from build123d import *

# Parameters (mm, degrees)
SKETCH3_R                   = 3.81
DOWELSUPPORT_DEPTH          = 1.27
SKETCH5_W                   = 6.35
SKETCH5_H                   = 44.45
SLIDERDOWELSUPPORT_DEPTH    = 1.27
LATERALSUPPORT_DEPTH        = 1.27
SKETCH8_W                   = 6.35
SKETCH8_H                   = 3
TABSUPPORT_DEPTH            = 1.27
STRINGDOWELSUPPORT_START    = -1.27
STRINGDOWELSUPPORT_DEPTH    = 5.08
INTERSUPPORT_DEPTH          = 1.27
SKETCH10_W                  = 6.35
SKETCH10_H                  = 3
TABBASE_DEPTH               = 1.27
SKETCH12_W                  = 6.35
SKETCH12_H                  = 3
TABDRAFT_DEPTH              = 1.73
TABDRAFT_DRAFT              = 5
TABDRAFT_PROFILE_2_DEPTH    = 1.73
TABDRAFT_PROFILE_2_DRAFT    = 5
STRINGDOWELHOLES_DEPTH      = 48.469574456
STRINGDOWELHOLES_DEPTH_BACK = 1.524
SKETCH14_R                  = 1.690500048
PULLEYDOWELHOLE_DEPTH       = 2.54


with BuildPart() as part:
    # Sketch3 → DowelSupport (new, symmetric)
    with BuildSketch(Plane(origin=(0, 0, 0), x_dir=(0, 0, -1), z_dir=(1, 0, 0))):
        with Locations((0, 37.30625)):
            Circle(SKETCH3_R)
    extrude(amount=DOWELSUPPORT_DEPTH, both=True)

    # Sketch8 → TabSupport (add, symmetric)
    with BuildSketch(Plane(origin=(0, 0, 0), x_dir=(0, 0, -1), z_dir=(1, 0, 0))):
        with Locations((0, 34.29)):
            Rectangle(SKETCH8_W, SKETCH8_H)
        with Locations((-12.7, 34.29)):
            Rectangle(SKETCH8_W, SKETCH8_H)
    extrude(amount=TABSUPPORT_DEPTH, both=True)


with BuildPart() as body_2:
    # Sketch5 → SliderDowelSupport (new, symmetric)
    with BuildSketch(Plane(origin=(0, 0, 0), x_dir=(0, 0, -1), z_dir=(1, 0, 0))):
        Rectangle(SKETCH5_W, SKETCH5_H)
    extrude(amount=SLIDERDOWELSUPPORT_DEPTH, both=True)



with BuildPart() as body_3:
    # Sketch6 → LateralSupport (new, symmetric)
    with BuildSketch(Plane(origin=(0, 0, 0), x_dir=(0, 0, -1), z_dir=(1, 0, 0))):
        Polygon((7.392863577, 39.741434671), (5.805363577, 42.491065329), (8.403439788, 43.991065329), (9.990939788, 41.241434671), align=None)
    extrude(amount=LATERALSUPPORT_DEPTH, both=True)


with BuildPart() as tabsupport_piece_1:
    # of the separate pieces the step leaves, piece 1, a body of its own (tabsupport_pieces)
    add(part.part.solids().sort_by_distance((1.27, 35.200193258, 3.175))[0])


with BuildPart() as tabsupport_piece_2:
    # of the separate pieces the step leaves, piece 2, a body of its own (tabsupport_pieces)
    add(part.part.solids().sort_by_distance((-1.27, 32.79, 9.525))[0])

    # Sketch15 → StringDowelSupport (add)
    with BuildSketch(Plane(origin=(0, 0, 0), x_dir=(0, 0, -1), z_dir=(1, 0, 0)).offset(STRINGDOWELSUPPORT_START)):
        with BuildLine():
            Line((-14.4145, 36.298), (-10.9855, 36.298))
            ThreePointArc((-10.9855, 36.298), (-8.4455, 33.758), (-10.9855, 31.218))
            Line((-10.9855, 31.218), (-14.4145, 31.218))
            ThreePointArc((-14.4145, 31.218), (-16.9545, 33.758), (-14.4145, 36.298))
        make_face()
    extrude(amount=STRINGDOWELSUPPORT_DEPTH)


with BuildPart() as body_2_1:
    add(body_2.part)

    add(body_3.part)  # InterSupport merges body 3

    add(tabsupport_piece_1.part)  # InterSupport merges TabSupport piece 1

    add(tabsupport_piece_2.part)  # InterSupport merges TabSupport piece 2
    # Sketch7 → InterSupport (add, symmetric)
    with BuildSketch(Plane(origin=(0, 0, 0), x_dir=(0, 0, -1), z_dir=(1, 0, 0))):
        Polygon((-15.691284512, 32.81461378), (-3.175, 15.875), (-3.175, 22.225), (3.175, 22.225), (3.175, 32.79), (0.989321966, 34.625476176), (-0.989321966, 39.987023824), (-10.9855, 36.298), (-14.4145, 36.298), align=None)
        Polygon((5.170363577, 43.590917591), (8.027863577, 38.641582409), (1.42875, 34.831582409), (-1.42875, 39.780917591), align=None)
    extrude(amount=INTERSUPPORT_DEPTH, both=True)

    # Sketch10 → TabBase (add)
    with BuildSketch(Plane.ZY.offset(1.27)):
        with Locations((0, 34.29)):
            Rectangle(SKETCH10_W, SKETCH10_H)
        with Locations((12.7, 34.29)):
            Rectangle(SKETCH10_W, SKETCH10_H)
    extrude(amount=TABBASE_DEPTH)


with BuildPart() as tabdraft_tool:
    # Sketch12 → TabDraft (with draft: the straight prism first)
    with BuildSketch(Plane.ZY.offset(2.54)):
        with Locations((0, 34.29)):
            Rectangle(SKETCH12_W, SKETCH12_H)
    extrude(amount=TABDRAFT_DEPTH)
    # TabDraft: the draft: its side faces are tilted about the plane it starts from
    tabdraft_sides = [tabdraft_tool.faces().sort_by_distance(p)[0] for p in [
        (-3.405, 34.29, 3.175),
        (-3.405, 35.79, 0),
        (-3.405, 34.29, -3.175),
        (-3.405, 32.79, 0),
    ]]
    draft(tabdraft_sides, Plane.ZY.offset(2.54), TABDRAFT_DRAFT)


with BuildPart() as body_2_2:
    add(body_2_1.part)

    # TabDraft: add tabdraft_tool
    add(tabdraft_tool.part)


with BuildPart() as tabdraft_profile_2_tool:
    # Sketch12 → TabDraft profile 2 (with draft: the straight prism first)
    with BuildSketch(Plane.ZY.offset(2.54)):
        with Locations((12.7, 34.29)):
            Rectangle(SKETCH12_W, SKETCH12_H)
    extrude(amount=TABDRAFT_PROFILE_2_DEPTH)
    # TabDraft profile 2: the draft: its side faces are tilted about the plane it starts from
    tabdraft_profile_2_sides = [tabdraft_profile_2_tool.faces().sort_by_distance(p)[0] for p in [
        (-3.405, 34.29, 9.525),
        (-3.405, 32.79, 12.7),
        (-3.405, 34.29, 15.875),
        (-3.405, 35.79, 12.7),
    ]]
    draft(tabdraft_profile_2_sides, Plane.ZY.offset(2.54), TABDRAFT_PROFILE_2_DRAFT)


with BuildPart() as body_2_3:
    add(body_2_2.part)

    # TabDraft profile 2: add tabdraft_profile_2_tool
    add(tabdraft_profile_2_tool.part)

    # Sketch16 → StringDowelHoles (cut, two sides: drawn at the far end of the back side and taken through both)
    with BuildSketch(Plane(origin=(1.27, 0, 0), x_dir=(0, 0, -1), z_dir=(1, 0, 0)).offset(-STRINGDOWELHOLES_DEPTH_BACK)):
        with BuildLine():
            Line((-12.905478326, 32.996), (-12.494521674, 32.996))
            ThreePointArc((-12.494521674, 32.996), (-9.294999952, 33.758), (-12.494521674, 34.52))
            Line((-12.494521674, 34.52), (-12.905478326, 34.52))
            ThreePointArc((-12.905478326, 34.52), (-16.105000048, 33.758), (-12.905478326, 32.996))
        make_face()
    extrude(amount=STRINGDOWELHOLES_DEPTH + STRINGDOWELHOLES_DEPTH_BACK, mode=Mode.SUBTRACT)

    # Sketch14 → PulleyDowelHole (cut)
    with BuildSketch(Plane(origin=(1.27, 0, 0), x_dir=(0, 0, -1), z_dir=(1, 0, 0))):
        with Locations((0, 37.30625)):
            Circle(SKETCH14_R)
    extrude(amount=-PULLEYDOWELHOLE_DEPTH, mode=Mode.SUBTRACT)

    # Mirror1: body 2 across plane


with BuildPart() as body_2_4:
    add(body_2_3.part)
    add(body_2_3.part.mirror(Plane.ZX))


solid = body_2_4.part
Design review of the part built by this model. Coordinates are the model's own, in mm. A direction names the side the tool comes from. Round coordinates to 2 decimals unless told otherwise and drop trailing zeros. Write each loop counter-clockwise with the first axis right and the second up, starting at its lowest first coordinate (ties: lowest second). Pieces come first, ordered by that corner, then holes. Notation, with made-up numbers: (-39.75, -6.75) - (11.25, -6.75) arc R11 ccw to (11.25, -0.75) - close; hole circle Ø4 at (11, 5). An arc over 180 degrees is marked (long way). Use a Markdown table: item, result. Add a question column.
1. We need section D-D (y = 12.5). State the section outline as (x, z) points (3 decimals).
2. We need section A-A (x = 2.25). State the section outline as (y, z) points.
3. We need section B-B (z = 0). State the section outline as (x, y) points.
4. Clearance check with flat-ended pins moving along their axes: pin 1 (0.6 mm diameter, centred on x = -2, y = -34.5, fed in from +Z) (3 decimals); pin 2 (3 mm diameter, centred on x = 0, y = 7.5, fed in from +Z) (3 decimals); pin 3 (1 mm diameter, centred on x = -2, z = 12, fed in from -Y). State where each tip first meets the part, or that it passes through.
5. For faces 1 (the face through (-3.393, -32.865, 12.656)), 2 (the face through (3, -31.218, 13)), 3 (the face through (0.02, -40.5, -8.71)), 4 (the face through (-3.4, -34.3, 3.1)), 5 (the face through (0.02, 23.65, 8.92)), list the 3-axis set-ups (+Z, -Z, +X, -X, +Y, -Y) from which the entire face can be reached by the end or side of a thin tool; tool diameter is ignored.
6. Mouldability with a two-part tool opening along Z and no side actions: class faces 6 (the face through (1.75, 33.821, 16.104)), 7 (the face through (-3.4, -34.3, 9.6)), 8 (the face through (-3.393, 32.865, 12.656)), 9 (the face through (2.522, -33.814, 8.446)) as +Z half, -Z half, draft (parallel to the pull), parting line (faces both ways), or undercut.
7. Wall thickness on probe 1 along Y at (x, z) = (0.3, 0); probe 2 along Z at (x, y) = (-2.75, -34); probe 3 along X at (y, z) = (27.5, -2): over which ranges is each line inside the solid? List them lowest first.
8. We need section C-C (z = 4.75). State the section outline as (x, y) points.
Output:
| question | item | result |
|---|---|---|
| 1 | outline | (-1.27, -3.175) - (1.27, -3.175) - (1.27, 3.175) - (-1.27, 3.175) - close |
| 2 | outline | (-36.3, 10.99) arc R2.54 ccw to (-31.22, 10.99) - (-31.22, 14.41) arc R2.54 ccw to (-36.3, 14.41) - close; (31.22, 10.99) arc R2.54 ccw to (36.3, 10.99) - (36.3, 14.41) arc R2.54 ccw to (31.22, 14.41) - close; hole (-34.52, 12.49) arc R1.69 ccw (long way) to (-33, 12.49) - (-33, 12.91) arc R1.69 ccw (long way) to (-34.52, 12.91) - close; hole (33, 12.49) arc R1.69 ccw (long way) to (34.52, 12.49) - (34.52, 12.91) arc R1.69 ccw (long way) to (33, 12.91) - close |
| 3 | outline | (-4.27, -35.64) - (-2.54, -35.79) - (-1.27, -35.79) - (-1.27, -35.62) - (1.27, -35.62) - (1.27, 35.62) - (-1.27, 35.62) - (-1.27, 35.79) - (-2.54, 35.79) - (-4.27, 35.64) - (-4.27, 32.94) - (-2.54, 32.79) - (-1.27, 32.79) - (-1.27, -32.79) - (-2.54, -32.79) - (-4.27, -32.94) - close; (-1.27, -41.12) - (1.27, -41.12) - (1.27, -39) - (-1.27, -39) - close; (-1.27, 39) - (1.27, 39) - (1.27, 41.12) - (-1.27, 41.12) - close |
| 4 | pin 1 | stops at z = 15.875 |
| 4 | pin 2 | stops at z = 3.175 |
| 4 | pin 3 | stops at y = -35.79 |
| 5 | face 1 | +Z, -Z, -X |
| 5 | face 2 | +Z, -Z, +X |
| 5 | face 3 | -Z, +X, -X |
| 5 | face 4 | -X, +Y, -Y |
| 5 | face 5 | +Z, +X, -X |
| 6 | face 6 | undercut |
| 6 | face 7 | undercut |
| 6 | face 8 | draft |
| 6 | face 9 | -Z half |
| 7 | probe 1 | y = -41.12 to -39, -35.62 to 35.62, 39 to 41.12 |
| 7 | probe 2 | z = -3.16 to 3.16, 9.54 to 15.86 |
| 7 | probe 3 | x = -1.27 to 1.27 |
| 8 | outline | (-1.27, -38.6) - (1.27, -38.6) - (1.27, -18.01) - (-1.27, -18.01) - close; (-1.27, 18.01) - (1.27, 18.01) - (1.27, 38.6) - (-1.27, 38.6) - close |
